```python
from build123d import *

# Parameters (mm, degrees)
F1_DEPTH = 4


with BuildPart() as f1:
    # F0 (on Top) → F1 (new body)
    with BuildSketch(Plane.XY):
        with BuildLine():
            Line((28.5, 6.5), (-28.5, 6.5))
            ThreePointArc((-28.5, 6.5), (-39.177078, 7.253738), (-49.642375, 9.5))
            Line((-49.642375, 9.5), (-82.5, 9.5))
            Line((-82.5, 9.5), (-82.5, -9.5))
            Line((-82.5, -9.5), (-49.642375, -9.5))
            ThreePointArc((-49.642375, -9.5), (-39.177078, -7.253738), (-28.5, -6.5))
            Line((-28.5, -6.5), (28.5, -6.5))
            ThreePointArc((28.5, -6.5), (39.177078, -7.253738), (49.642375, -9.5))
            Line((49.642375, -9.5), (82.5, -9.5))
            Line((82.5, -9.5), (82.5, 9.5))
            Line((82.5, 9.5), (49.642375, 9.5))
            ThreePointArc((49.642375, 9.5), (39.177078, 7.253738), (28.5, 6.5))
        make_face()
    extrude(amount=F1_DEPTH)


solid = f1.part
```
Geometry check sheet. Reference: the model listing, model coordinates, mm. A direction names the side the tool comes from. Round coordinates to 2 decimals unless told otherwise and drop trailing zeros. Loops run counter-clockwise (first coordinate to the right, second up) from the corner with the lowest first, then second, coordinate; pieces in that order, holes last. Notation, with made-up numbers: (44, -34.75) - (85, -34.75) arc R30 ccw to (85, -2.75) - close; hole circle Ø1 at (24.25, 22.5). An arc over 180 degrees is marked (long way). Write item = value, one per line. Start each with the question number.
1. Set-up check for faces 5 (the face through (39.029, -7.233, 1.972)), 6 (the face through (-66, -9.5, 2)), 7 (the face through (-39.029, 7.233, 1.972)): record each of +Z, -Z, +X, -X, +Y, -Y from which the full face is reachable in a straight line by a thin tool's end or side.
2. Depth check by flat-ended pin: pin 1 (1.5 mm diameter, centred on x = 17.5, z = 1, fed in from +Y). Enter the tip coordinate at first touch or a pass-through.
3. Mould release check, pull along X, two halves, no side actions. Record for faces 1 (the face through (0, -6.5, 2)), 2 (the face through (-82.5, 0, 2)), 3 (the face through (-39.326, -7.275, 1.972)), 4 (the face through (-66, 9.5, 2)): released by +X, released by -X, zero draft, split by the parting line, or undercut.
4. Section check B-B on y = 8. Enter the section's corners in (x, z), then the cut area to 3 significant figures.
5. Section check A-A on z = 1.1. Enter the section's corners in (x, y), then the cut area to 3 significant figures.
6. Section check C-C on x = -5.5. Enter the section's corners in (y, z), then the cut area to 3 significant figures.
7. Thickness scan on line 1 (Y direction, x = 5, z = 3.3); line 2 (Y direction, x = -39, z = 2.8). Record the ranges inside material, lowest first.
Working result:
q1.face_5 = +Z, -Z, -Y
q1.face_6 = +Z, -Z, +X, -X, -Y
q1.face_7 = +Z, -Z, +Y
q2.pin_1 = 6.5
q3.face_1 = undercut
q3.face_2 = released by -X
q3.face_3 = undercut
q3.face_4 = zero draft
q4.outline = (-82.5, 0) - (-43.52, 0) - (-43.52, 4) - (-82.5, 4) - close; (43.52, 0) - (82.5, 0) - (82.5, 4) - (43.52, 4) - close
q4.area = 312 mm^2
q5.outline = (-82.5, -9.5) - (-49.64, -9.5) arc R76 cw to (-28.5, -6.5) - (28.5, -6.5) arc R76 cw to (49.64, -9.5) - (82.5, -9.5) - (82.5, 9.5) - (49.64, 9.5) arc R76 cw to (28.5, 6.5) - (-28.5, 6.5) arc R76 cw to (-49.64, 9.5) - (-82.5, 9.5) - close
q5.area = 2,620 mm^2
q6.outline = (-6.5, 0) - (6.5, 0) - (6.5, 4) - (-6.5, 4) - close
q6.area = 52.0 mm^2
q7.line_1 = -6.5 to 6.5
q7.line_2 = -7.23 to 7.23
